```python
from build123d import *

# Parameters (mm, degrees)
SKETCH4_W                = 200
SKETCH4_H                = 200
BOSS_EXTRUDE1_DEPTH      = 150
SKETCH6_W                = 196
SKETCH6_H                = 196
CUT_EXTRUDE1_DEPTH       = 2
SKETCH7_W                = 192
SKETCH7_H                = 192
CUT_EXTRUDE2_DEPTH       = 92
SKETCH9_W                = 28
SKETCH9_H                = 46.8
INLET_DEPTH              = 4
SKETCH13_W               = 4
SKETCH13_H               = 132
AIRFLOW_DEPTH            = 4
SKETCH11_W               = 25.2
SKETCH11_H               = 71.2
CUT_EXTRUDE5_DEPTH       = 4
SKETCH11_4_R             = 1.25
LCD_MOUNTING_DEPTH       = 4
SKETCH12_R               = 0.55
SKETCH12_R_2             = 1
POST_KNOB_MOUNTING_DEPTH = 4
SKETCH14_R               = 3
CUT_EXTRUDE10_DEPTH      = 56
SKETCH17_W               = 192
SKETCH17_H               = 192
CUT_EXTRUDE11_DEPTH      = 52
SKETCH18_R               = 1.6
CUT_EXTRUDE12_DEPTH      = 4
SKETCH20_W               = 15
SKETCH20_H               = 15
CUT_EXTRUDE13_DEPTH      = 4


with BuildPart() as part:
    # Sketch4 → Boss-Extrude1 (new body)
    with BuildSketch(Plane.XY):
        with Locations((100, 100)):
            Rectangle(SKETCH4_W, SKETCH4_H)
    extrude(amount=BOSS_EXTRUDE1_DEPTH)

    # Sketch6 → Cut-Extrude1 (cut)
    with BuildSketch(Plane.XY.offset(150)):
        with Locations((100, 100)):
            Rectangle(SKETCH6_W, SKETCH6_H)
    extrude(amount=-CUT_EXTRUDE1_DEPTH, mode=Mode.SUBTRACT)

    # Sketch7 → Cut-Extrude2 (cut)
    with BuildSketch(Plane.XY.offset(148)):
        with Locations((100, 100)):
            Rectangle(SKETCH7_W, SKETCH7_H)
    extrude(amount=-CUT_EXTRUDE2_DEPTH, mode=Mode.SUBTRACT)

    # Sketch9 → Inlet (cut)
    with BuildSketch(Plane(origin=(200, 0, 0), x_dir=(0, 0, -1), z_dir=(1, 0, 0))):
        with Locations((-61, 27.4)):
            Rectangle(SKETCH9_W, SKETCH9_H)
    extrude(amount=-INLET_DEPTH, mode=Mode.SUBTRACT)

    # Sketch13 → Airflow (cut)
    with BuildSketch(Plane(origin=(200, 0, 0), x_dir=(0, 0, -1), z_dir=(1, 0, 0))):
        with Locations((-10, 126)):
            Rectangle(SKETCH13_W, SKETCH13_H)
        with Locations((-20, 126)):
            Rectangle(SKETCH13_W, SKETCH13_H)
        with Locations((-30, 126)):
            Rectangle(SKETCH13_W, SKETCH13_H)
        with Locations((-40, 126)):
            Rectangle(SKETCH13_W, SKETCH13_H)
        with Locations((-50, 126)):
            Rectangle(SKETCH13_W, SKETCH13_H)
        with Locations((-60, 126)):
            Rectangle(SKETCH13_W, SKETCH13_H)
        with Locations((-70, 126)):
            Rectangle(SKETCH13_W, SKETCH13_H)
        with Locations((-80, 126)):
            Rectangle(SKETCH13_W, SKETCH13_H)
        with Locations((-90, 126)):
            Rectangle(SKETCH13_W, SKETCH13_H)
        with Locations((-100, 126)):
            Rectangle(SKETCH13_W, SKETCH13_H)
        with Locations((-110, 126)):
            Rectangle(SKETCH13_W, SKETCH13_H)
        with Locations((-120, 126)):
            Rectangle(SKETCH13_W, SKETCH13_H)
        with Locations((-130, 126)):
            Rectangle(SKETCH13_W, SKETCH13_H)
        with Locations((-140, 126)):
            Rectangle(SKETCH13_W, SKETCH13_H)
    extrude(amount=-AIRFLOW_DEPTH, mode=Mode.SUBTRACT)

    # Sketch11 → Cut-Extrude5 (cut)
    with BuildSketch(Plane.ZY):
        with Locations((112.5, 100)):
            Rectangle(SKETCH11_W, SKETCH11_H)
    extrude(amount=-CUT_EXTRUDE5_DEPTH, mode=Mode.SUBTRACT)

    # Sketch11<4> → LCD/Mounting (cut)
    with BuildSketch(Plane.ZY):
        with Locations((128, 137.5)):
            Circle(SKETCH11_4_R)
        with Locations((97, 137.5)):
            Circle(SKETCH11_4_R)
        with Locations((97, 62.5)):
            Circle(SKETCH11_4_R)
        with Locations((128, 62.5)):
            Circle(SKETCH11_4_R)
    extrude(amount=-LCD_MOUNTING_DEPTH, mode=Mode.SUBTRACT)

    # Sketch12 → Post/Knob Mounting (cut)
    with BuildSketch(Plane.ZY):
        with Locations((37.5, 100)):
            Circle(SKETCH12_R)
        with Locations((37.5, 80)):
            Circle(SKETCH12_R)
        with Locations((37.5, 60)):
            Circle(SKETCH12_R)
        with Locations((37.5, 148)):
            Circle(SKETCH12_R_2)
    extrude(amount=-POST_KNOB_MOUNTING_DEPTH, mode=Mode.SUBTRACT)

    # Sketch14 → Cut-Extrude10 (cut)
    with BuildSketch(Plane.XY.offset(56)):
        with Locations((37.506, 103.996)):
            Circle(SKETCH14_R)
        with Locations((171.555, 104.25)):
            Circle(SKETCH14_R)
        with Locations((36.935, 13.318)):
            Circle(SKETCH14_R)
        with Locations((171.555, 13.318)):
            Circle(SKETCH14_R)
    extrude(amount=-CUT_EXTRUDE10_DEPTH, mode=Mode.SUBTRACT)

    # Sketch17 → Cut-Extrude11 (cut)
    with BuildSketch(Plane.XY.offset(56)):
        with Locations((100, 100)):
            Rectangle(SKETCH17_W, SKETCH17_H)
    extrude(amount=-CUT_EXTRUDE11_DEPTH, mode=Mode.SUBTRACT)

    # Sketch18 → Cut-Extrude12 (cut)
    with BuildSketch(Plane.XY.offset(4)):
        with Locations((126.8, 188.46)):
            Circle(SKETCH18_R)
        with Locations((126.8, 142.74)):
            Circle(SKETCH18_R)
        with Locations((76, 157.98)):
            Circle(SKETCH18_R)
        with Locations((76, 185.92)):
            Circle(SKETCH18_R)
    extrude(amount=-CUT_EXTRUDE12_DEPTH, mode=Mode.SUBTRACT)

    # Sketch20 → Cut-Extrude13 (cut)
    with BuildSketch(Plane(origin=(0, 200, 0), x_dir=(1, 0, 0), z_dir=(0, 1, 0))):
        with Locations((175, -36)):
            Rectangle(SKETCH20_W, SKETCH20_H)
    extrude(amount=-CUT_EXTRUDE13_DEPTH, mode=Mode.SUBTRACT)


solid = part.part
```
Could you check a few things on this model? Use its own coordinates, in mm. A direction names the side the tool comes from. Round coordinates to 2 decimals unless told otherwise and drop trailing zeros. Write each loop counter-clockwise with the first axis right and the second up, starting at its lowest first coordinate (ties: lowest second). Pieces come first, ordered by that corner, then holes.
(1) Thinking about a two-plate mould opening in X: for faces 3 (the face through (169.174, 102.425, 2.028)), 4 (the face through (200, 99, 74)), 5 (the face through (0, 99, 74)), which applies, +X half, -X half, draft (parallel to the pull), parting line (faces both ways), or undercut?
Findings below:
face 3: undercut
face 4: +X half
face 5: -X half
(2) Suppose I cut it at A-A on y = 22. Write out the boundary of the cut face in (x, z).
Findings below:
outline: (0, 0) - (200, 0) - (200, 47) - (196, 47) - (196, 4) - (4, 4) - (4, 148) - (2, 148) - (2, 150) - (0, 150) - close; (196, 75) - (200, 75) - (200, 150) - (198, 150) - (198, 148) - (196, 148) - close
(3) If I drill on probe 1 along Y at (x, z) = (1.6, 97); probe 2 along Y at (x, z) = (105, 107); probe 3 along Z at (x, y) = (1.05, 137.5), over which ranges is the centre line in solid material (lowest first)?
Findings below:
probe 1: y = 0 to 61.25, 63.75 to 136.25, 138.75 to 200
probe 2: y = 0 to 4, 196 to 200
probe 3: z = 0 to 95.75, 98.25 to 126.75, 129.25 to 150
(4) Which directions (+Z, -Z, +X, -X, +Y, -Y) give clear straight access to the entire face, cutting with the end or side of a thin tool? Please do faces 1 (the face through (36.28, 10.39, 2.03)), 2 (the face through (99, 196, 77)).
Findings below:
face 1: +Z, -Z
face 2: +Z
(5) Suppose I cut it at B-B on x = 45.5. Write out the boundary of the cut face in (y, z), and give its area (3 significant figures).
Findings below:
outline: (0, 0) - (200, 0) - (200, 150) - (198, 150) - (198, 148) - (196, 148) - (196, 4) - (4, 4) - (4, 148) - (2, 148) - (2, 150) - (0, 150) - close
area: 1,960 mm2
(6) Suppose I cut it at C-C on y = 95. State how many separate pieces and enclosed holes the cut face has, and give its area (3 significant figures).
Findings below:
separate pieces: 16
enclosed holes: 0
area: 1,640 mm2
(7) For pin 1 (5 mm diameter, centred on x = 36.935, y = 13.318, fed in from -Z); pin 2 (5 mm diameter, centred on x = 150, y = 111.5, fed in from +Z), each with a flat end and sliding along its axis, tell me the tip position at first contact or that it passes through.
Findings below:
pin 1: passes through
pin 2: stops at z = 4
